```python
from build123d import *

# Parameters (mm, degrees)
F1_DEPTH = 5


with BuildPart() as f1:
    # F0 (on Top) → F1 (new body)
    with BuildSketch(Plane.XY):
        Polygon((5, 0), (0, 0), (0, -30), (360, -30), (360, 0), (355, 0), (355, -27), (241.666667, -27), (241.666667, 0), (236.666667, 0), (236.666667, -27), (123.333333, -27), (123.333333, 0), (118.333333, 0), (118.333333, -27), (5, -27), align=None)
    extrude(amount=F1_DEPTH)

    # F2: F1 across face


with BuildPart() as f1_1:
    add(f1.part)
    add(f1.part.mirror(Plane(origin=(2.5, 0, 2.5), x_dir=(-1, 0, 0), z_dir=(0, 1, 0))))


solid = f1_1.part
```
Design review of the part built by this model. Coordinates are the model's own, in mm. Round coordinates to 2 decimals unless told otherwise and drop trailing zeros. Order: outer loops, then holes, each group sorted by start corner. A loop starts at its lowest first (then second) coordinate and runs counter-clockwise, first axis right, second up. Notation, with made-up numbers: (0.25, -1) - (42.25, -1) arc R11 ccw to (42.25, 8) - close; hole circle Ø7 at (25.5, 47.25). An arc over 180 degrees is marked (long way). One line per question, with ' | ' between items.
Item 1: Wall thickness on line 1 (X direction, y = -18.5, z = 2.8); line 2 (Y direction, x = 52, z = 2.5): over which ranges is each line inside the solid? List them lowest first. Write a range as [from, to].
Checks:
line 1: [0, 5], [118.33, 123.33], [236.67, 241.67], [355, 360] | line 2: [-30, -27], [27, 30]
Item 2: Take a section at C-C, the plane x = 186. Write out the cut boundary in (y, z), then the cut area to 3 significant figures.
Checks:
outline: (-30, 0) - (-27, 0) - (-27, 5) - (-30, 5) - close; (27, 0) - (30, 0) - (30, 5) - (27, 5) - close | area: 30.0 mm²
Item 3: Take a section at B-B, the plane z = 3.5. Write out the cut boundary in (x, y).
Checks:
outline: (0, -30) - (360, -30) - (360, 30) - (0, 30) - close; hole (5, -27) - (118.33, -27) - (118.33, 27) - (5, 27) - close; hole (123.33, -27) - (236.67, -27) - (236.67, 27) - (123.33, 27) - close; hole (241.67, -27) - (355, -27) - (355, 27) - (241.67, 27) - close
Item 4: Take a section at A-A, the plane y = -19.5. Write out the cut boundary in (x, z).
Checks:
outline: (0, 0) - (5, 0) - (5, 5) - (0, 5) - close; (118.33, 0) - (123.33, 0) - (123.33, 5) - (118.33, 5) - close; (236.67, 0) - (241.67, 0) - (241.67, 5) - (236.67, 5) - close; (355, 0) - (360, 0) - (360, 5) - (355, 5) - close
